from build123d import *
from build123d import SkipClean  # not in build123d's __all__

# Parameters (mm, degrees)
F0_R     = 42.2654661293
F1_DEPTH = 101.6
F2_W     = 99.4848832185
F2_H     = 84.4806035552
F3_DEPTH = 12.7
F4_R     = 31.9997887228
F5_DEPTH = 101.601
F6_W     = 54.3876717536
F6_H     = 11.9783656307
F7_DEPTH = 101.6
F9_DEPTH = 48.3780729043


with BuildPart() as f1:
    # F0 (on Top) → F1 (new body)
    with BuildSketch(Plane.XY):
        with Locations((62.4748729169, 0)):
            Circle(F0_R)
    extrude(amount=F1_DEPTH)

    # F2 (on face) → F3 (join)
    with BuildSketch(Plane(origin=(0, 0, 0), x_dir=(1, 0, 0), z_dir=(0, 0, -1))):
        with Locations((15.9839019028, -0.1000886066)):
            Rectangle(F2_W, F2_H)
    extrude(amount=-F3_DEPTH)

    # F4 (on face) → F5 (cut, through all)
    with BuildSketch(Plane.XY.offset(101.6)):
        with Locations((62.4748729169, 0)):
            Circle(F4_R)
    extrude(amount=-F5_DEPTH, mode=Mode.SUBTRACT)

    # F6 (on face) → F7 (join)
    with BuildSketch(Plane.XY.offset(12.7)):
        with Locations((-6.5647038297, -0.0474997047)):
            Rectangle(F6_W, F6_H)
    with SkipClean():  # cleaning this boolean's faces spoils the solid; the shape is the same uncleaned
        extrude(amount=F7_DEPTH)

    # F8 (on face) → F9 (cut, through all)
    with BuildSketch(Plane.XZ.offset(6.0366825201)):
        Polygon((-33.7585397065, 13.207843317), (20.6291320471, 100.9798197685), (20.6291320471, 114.3), (-33.7585397065, 114.3), align=None)
    with SkipClean():  # cleaning this boolean's faces spoils the solid; the shape is the same uncleaned
        extrude(amount=-F9_DEPTH, mode=Mode.SUBTRACT)


solid = f1.part
For this review, take the finished solid that the model builds, in its own axes (mm). A direction names the side the tool comes from. Round coordinates to 2 decimals unless told otherwise and drop trailing zeros. Order: outer loops, then holes, each group sorted by start corner. A loop starts at its lowest first (then second) coordinate and runs counter-clockwise, first axis right, second up. Notation, with made-up numbers: (59, -5.75) -> (101, -5.75) arc R22 cw to (101, 10.25) -> close; hole circle Ø6 at (15.5, -10). An arc over 180 degrees is marked (long way). Write item = value, one per line. Start each with the question number.
1) Take a section at D-D on x = -14.5. State the section outline as (y, z) points, plus the area to 3 significant figures.
2) Take a section at B-B on y = -25. State the section outline as (x, z) points, plus the area to 3 significant figures.
3) Take a section at A-A on x = 85.5. State the section outline as (y, z) points.
4) Take a section at C-C on z = 50. State the section outline as (x, y) points, plus the area to 3 significant figures.
5) Tool access review of faces 4 (the face through (-1, 5.942, 46)), 5 (the face through (-6.945, -0.131, 56.479)), 6 (the face through (12, -42.14, 6)): name each direction out of +Z, -Z, +X, -X, +Y, -Y from which nothing blocks a thin tool from reaching the whole face with its end or side.
6) Insertion check: pin 1 (6 mm diameter, centred on x = -17, y = -18.5, fed in from -Z); pin 2 (6.5 mm diameter, centred on x = 35, z = 8.5, fed in from -Y); pin 3 (1 mm diameter, centred on y = -19.5, z = 84.5, fed in from +X); pin 4 (10 mm diameter, centred on x = 86.5, z = 66, fed in from +Y). Each pin has a flat end and moves straight along its axis. Give the tip position at first contact, or say it passes through.
7) The part is to be moulded in two halves that separate along Y. For faces 1 (the face through (-1, -6.037, 46)), 2 (the face through (92.035, -12.256, 51.511)), 3 (the face through (2, -24, 12.7)), say which applies: +Y half, -Y half, draft (parallel to the pull), parting line (faces both ways), or undercut.
8) To check wall thickness, follow line 1 (Z direction, x = 17, y = 12.5); line 2 (X direction, y = -11, z = 40); line 3 (Y direction, x = 44, z = 79.5). State the ranges of each line that lie inside material, in increasing order. Write a range as from..to.
Verdict:
q1.outline = (-42.14, 0) -> (42.34, 0) -> (42.34, 12.7) -> (5.94, 12.7) -> (5.94, 44.29) -> (-6.04, 44.29) -> (-6.04, 12.7) -> (-42.14, 12.7) -> close
q1.area = 1,450 mm2
q2.outline = (-33.76, 0) -> (42.5, 0) -> (42.5, 101.6) -> (28.4, 101.6) -> (28.4, 12.7) -> (-33.76, 12.7) -> close; (82.45, 0) -> (96.55, 0) -> (96.55, 101.6) -> (82.45, 101.6) -> close
q2.area = 3,660 mm2
q3.outline = (-35.44, 0) -> (-22.22, 0) -> (-22.22, 101.6) -> (-35.44, 101.6) -> close; (22.22, 0) -> (35.44, 0) -> (35.44, 101.6) -> (22.22, 101.6) -> close
q4.outline = (-10.96, -6.04) -> (20.63, -6.04) -> (20.63, -5.94) arc R42.27 ccw (long way) to (20.63, 5.94) -> (-10.96, 5.94) -> close; hole circle Ø64 at (62.47, 0)
q4.area = 2,770 mm2
q5.face_4 = +Z, -X, +Y
q5.face_5 = +Z, -X, +Y, -Y
q5.face_6 = +Z, -Z, -X, -Y
q6.pin_1 = 0
q6.pin_2 = -42.14
q6.pin_3 = 100.23
q6.pin_4 = 37.74
q7.face_1 = -Y half
q7.face_2 = undercut
q7.face_3 = draft
q8.line_1 = 0..12.7
q8.line_2 = 21.67..32.43, 92.52..103.28
q8.line_3 = -38.01..-26.13, 26.13..38.01
